Here's the drawing with two shaded views (mm, measured from the low corner). I have some questions. Round coordinates to 2 decimals unless told otherwise and drop trailing zeros. Loops run counter-clockwise (first coordinate to the right, second up) from the corner with the lowest first, then second, coordinate; pieces in that order, holes last. Notation, with made-up numbers: M 69.25,83 L 85.25,83 A24 ccw 85.25,103 Z; hole C 15,-35 d2. An arc over 180 degrees is marked long. One line per item, written item: value. Start each with the question number.
Q1. Imagine slicing it at D-D (x = 18). Please give me the cut outline in (y, z) (1 decimal), then the cut area to 3 significant figures.
Q2. Thinking about a two-plate mould opening in Y: for the marked faces 1, 2 and 3, which applies, released by +Y, released by -Y, zero draft, split by the parting line, or undercut?
Q3. Imagine slicing it at B-B (y = 23). Please give me the cut outline in (x, z) (1 decimal).
Q4. Please list where these lines run through material, in increasing order: line 1 along X through (y, z) = (27.5, 1.9) (1 decimal); line 2 along X through (y, z) = (11, 1.45) (1 decimal); line 3 along Y through (x, z) = (27, 2.6) (1 decimal).
Q5. I'm going to push a flat-ended pin straight in: pin 1 Ø1 at (x, z) = (26, 2.5) entering from +Y (1 decimal). Where does the tip first touch, or does it pass through?
Q6. Imagine slicing it at A-A (x = 28). Please give me the cut outline in (y, z) (1 decimal).
Q7. Imagine slicing it at C-C (z = 2.7). Give the number of separate pieces and of enclosed holes in the cut face, then the cut area to 3 significant figures.
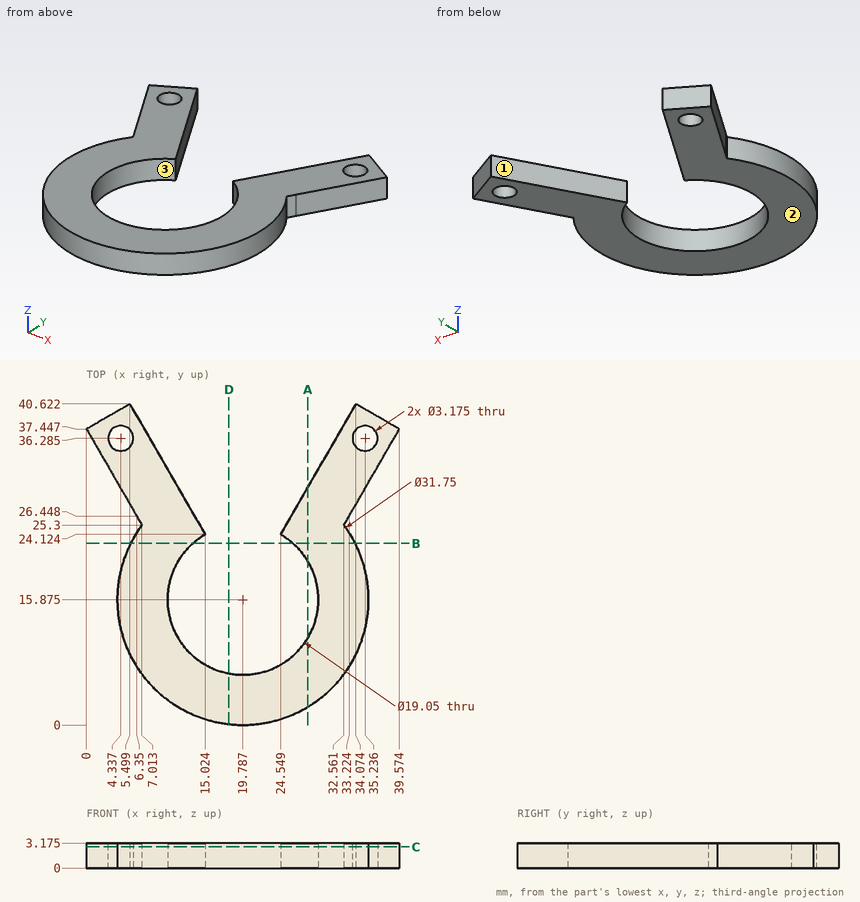
Report:
1. outline: M 0.1,0 L 6.5,0 L 6.5,3.2 L 0.1,3.2 Z
1. area: 20.4 mm²
2. face 1: released by +Y
2. face 2: zero draft
2. face 3: undercut
3. outline: M 5.6,0 L 13.5,0 L 13.5,3.2 L 5.6,3.2 Z; M 26.1,0 L 34,0 L 34,3.2 L 26.1,3.2 Z
4. line 1: x = 5.7 to 13.1, 26.5 to 33.8
4. line 2: x = 4.7 to 11.6, 28 to 34.9
4. line 3: y = 1.7 to 9.7, 22.1 to 28.4
5. pin 1: stops at y = 27.5
6. outline: M 2.3,0 L 11.1,0 L 11.1,3.2 L 2.3,3.2 Z; M 20.7,0 L 30.1,0 L 30.1,3.2 L 20.7,3.2 Z
7. separate pieces: 1
7. enclosed holes: 2
7. area: 573 mm²
